```python
from build123d import *

# Parameters (mm, degrees)
F0_W           = 42
F0_H           = 14
F1_DEPTH       = 6
F2_W           = 18
F2_H           = 14
F3_DEPTH       = 26.8
F6_D           = 4.4
F6_CSINK_D     = 8.96
F6_CSINK_ANGLE = 90
F7_D           = 8


with BuildPart() as f1:
    # F0 (on Top) → F1 (new body)
    with BuildSketch(Plane.XY):
        Rectangle(F0_W, F0_H)
    extrude(amount=F1_DEPTH)

    # F2 (on face) → F3 (join)
    with BuildSketch(Plane.XY.offset(6)):
        Rectangle(F2_W, F2_H)
    extrude(amount=F3_DEPTH)

    # F6 (through all)
    with Locations(Plane.XY.offset(6)):
        with Locations((-16, 0), (16, 0)):
            CounterSinkHole(F6_D / 2, F6_CSINK_D / 2, counter_sink_angle=F6_CSINK_ANGLE)

    # F7 (through all)
    with Locations(Plane.XZ.offset(7)):
        with Locations((0, 20)):
            Hole(F7_D / 2)


solid = f1.part
```
Source: CAD feature listing. Evaluate the final solid. Frame: model axes, mm. A direction names the side the tool comes from. Round coordinates to 2 decimals unless told otherwise and drop trailing zeros. Loops run counter-clockwise (first coordinate to the right, second up) from the corner with the lowest first, then second, coordinate; pieces in that order, holes last.
1. Mould query, pull axis Y, two halves, no side actions, for faces 4 (the cylindrical face through (13.968, -0.843, 1.834)), 5 (the flat face through (-11, 0, 6)), 6 (the flat face through (0, 7, 13)), 7 (the conical face through (-18.204, 0.694, 3.831)). Classes: released by +Y, released by -Y, zero draft, split by the parting line, or undercut.
2. Section query D-D on y = 5.75. Output: boundary loops of the cut face in (x, z).
3. Section query A-A on x = 0. Output: boundary loops of the cut face in (y, z).
4. Section query B-B on y = 0. Output: boundary loops of the cut face in (x, z).
5. Contact query for flat-ended pins moving along their axis: pin 1 (5.5 mm diameter, centred on x = 16, y = 0, fed in from +Z); pin 2 (3 mm diameter, centred on y = 5.5, z = 17, fed in from -X); pin 3 (3.5 mm diameter, centred on x = 17.5, y = 0, fed in from +Z); pin 4 (2.5 mm diameter, centred on x = -16, y = 0, fed in from -Z). Output: stop coordinate, or through.
6. Section query C-C on z = 19.5. Output: boundary loops of the cut face in (x, y).
7. Access query for faces 1 (the flat face through (-9, 0, 19)), 2 (the flat face through (9, 0, 19)), 3 (the cylindrical face through (-18.032, -0.843, 1.834)). Directions: +Z, -Z, +X, -X, +Y, -Y. A direction counts if a zero-diameter tool reaches every point of the face in a straight line with its end or side. Return the directions, or none.
8. Ray query, L1, parallel to X at y = 0, z = 2.3; L2, parallel to Y at x = -16, z = 1; L3, parallel to X at y = -5, z = 11. Return the intervals inside material, ascending.
Answers below:
1. face 4: undercut
1. face 5: zero draft
1. face 6: released by +Y
1. face 7: undercut
2. outline: (-21, 0) - (21, 0) - (21, 6) - (9, 6) - (9, 32.8) - (-9, 32.8) - (-9, 6) - (-21, 6) - close; hole circle Ø8 at (0, 20)
3. outline: (-7, 0) - (7, 0) - (7, 16) - (-7, 16) - close; (-7, 24) - (7, 24) - (7, 32.8) - (-7, 32.8) - close
4. outline: (-21, 0) - (-18.2, 0) - (-18.2, 3.72) - (-20.48, 6) - (-21, 6) - close; (-13.8, 0) - (13.8, 0) - (13.8, 3.72) - (11.52, 6) - (9, 6) - (9, 32.8) - (-9, 32.8) - (-9, 6) - (-11.52, 6) - (-13.8, 3.72) - close; (18.2, 0) - (21, 0) - (21, 6) - (20.48, 6) - (18.2, 3.72) - close; hole circle Ø8 at (0, 20)
5. pin 1: stops at z = 4.27
5. pin 2: stops at x = -9
5. pin 3: stops at z = 4.77
5. pin 4: passes through
6. outline: (-9, -7) - (-3.97, -7) - (-3.97, 7) - (-9, 7) - close; (3.97, -7) - (9, -7) - (9, 7) - (3.97, 7) - close
7. face 1: +Z, -X, +Y, -Y
7. face 2: +Z, +X, +Y, -Y
7. face 3: +Z, -Z
8. L1: x = -21 to -18.2, -13.8 to 13.8, 18.2 to 21
8. L2: y = -7 to -2.2, 2.2 to 7
8. L3: x = -9 to 9
